from build123d import *

# Parameters (mm, degrees)
SKETCH1_W           = 228.6
SKETCH1_H           = 228.6
SKETCH1_W_2         = 180.086
SKETCH1_H_2         = 180.086
BOSS_EXTRUDE1_DEPTH = 7.62
BOSS_EXTRUDE2_START = 7.62
SKETCH1_3_W         = 180.086
SKETCH1_3_H         = 180.086
BOSS_EXTRUDE2_DEPTH = 7.62


with BuildPart() as part:
    # Sketch1 → Boss-Extrude1 (new body)
    # profile 1 of 2: a face of its own
    with BuildSketch(Plane(origin=(0, 0, 0), x_dir=(0, 0, -1), z_dir=(1, 0, 0))):
        with Locations((114.3, -114.3)):
            Rectangle(SKETCH1_W, SKETCH1_H)
        with Locations((114.3, -114.3)):
            Rectangle(SKETCH1_W_2, SKETCH1_H_2, mode=Mode.SUBTRACT)
    # profile 2 of 2: a face of its own
    with BuildSketch(Plane(origin=(0, 0, 0), x_dir=(0, 0, -1), z_dir=(1, 0, 0))):
        with Locations((114.3, -114.3)):
            Rectangle(SKETCH1_W_2, SKETCH1_H_2)
    extrude(amount=BOSS_EXTRUDE1_DEPTH)

    # Sketch1<3> → Boss-Extrude2 (add)
    with BuildSketch(Plane(origin=(0, 0, 0), x_dir=(0, 0, -1), z_dir=(1, 0, 0)).offset(BOSS_EXTRUDE2_START)):
        with Locations((114.3, -114.3)):
            Rectangle(SKETCH1_3_W, SKETCH1_3_H)
    extrude(amount=BOSS_EXTRUDE2_DEPTH)


solid = part.part
Geometry: final body of the model. Coordinates: model frame, mm. A direction names the side the tool comes from. Give positions to 0.01 mm unless a question says otherwise; leave off trailing zeros. Loops run counter-clockwise (first coordinate to the right, second up) from the corner with the lowest first, then second, coordinate; pieces in that order, holes last. Notation, with made-up numbers: M 61,58.5 L 96,58.5 A20 cw 96,81.5 Z; hole C -28,75.5 d1. An arc over 180 degrees is marked long. Put each result on its own line as item: value.
1) Cut plane D-D, the plane z = -15.5. Return the cut outline in (x, y), plus the area to 3 significant figures.
Computed values:
outline: M 0,-228.6 L 7.62,-228.6 L 7.62,0 L 0,0 Z
area: 1,740 mm^2
2) Material intervals for L1, parallel to X at y = -134, z = -21; L2, parallel to Y at x = 12.5, z = -41.5, sorted ascending. Write a range as from..to.
Computed values:
L1: x = 0..7.62
L2: y = -204.34..-24.26
3) Cut plane C-C, the plane x = 11.25. Return the cut outline in (y, z), plus the area to 3 significant figures.
Computed values:
outline: M -204.34,-204.34 L -24.26,-204.34 L -24.26,-24.26 L -204.34,-24.26 Z
area: 32,400 mm^2
4) Reachability of faces 1 (the flat face through (11, -116, -24.257)), 2 (the flat face through (11, -24.257, -113)), 3 (the flat face through (4, -228.6, -113)), 4 (the flat face through (11, -204.343, -113)), 5 (the flat face through (11, -116, -204.343)) from +Z, -Z, +X, -X, +Y, -Y: full face, straight path, thin tool, end or side. Return the list, or none.
Computed values:
face 1: +Z, +X, +Y, -Y
face 2: +Z, -Z, +X, +Y
face 3: +Z, -Z, +X, -X, -Y
face 4: +Z, -Z, +X, -Y
face 5: -Z, +X, +Y, -Y
5) First-contact query: P1, Ø4, axis at x = 9.5, z = -156.5, coming from the +Y side; P2, Ø2, axis at x = 9.5, z = -74.5, coming from the +Y side; P3, Ø2.5, axis at x = 13, z = -78.5, coming from the -Y side; P4, Ø4, axis at x = 11, y = -90, coming from the -Z side. Flat tips, straight axial feed; report the tip coordinate or a pass-through.
Computed values:
P1: stops at y = 0
P2: stops at y = -24.26
P3: stops at y = -204.34
P4: stops at z = -204.34
6) Cut plane A-A, the plane z = -96. Return the cut outline in (x, y), plus the area to 3 significant figures.
Computed values:
outline: M 0,-228.6 L 7.62,-228.6 L 7.62,-204.34 L 15.24,-204.34 L 15.24,-24.26 L 7.62,-24.26 L 7.62,0 L 0,0 Z
area: 3,110 mm^2
